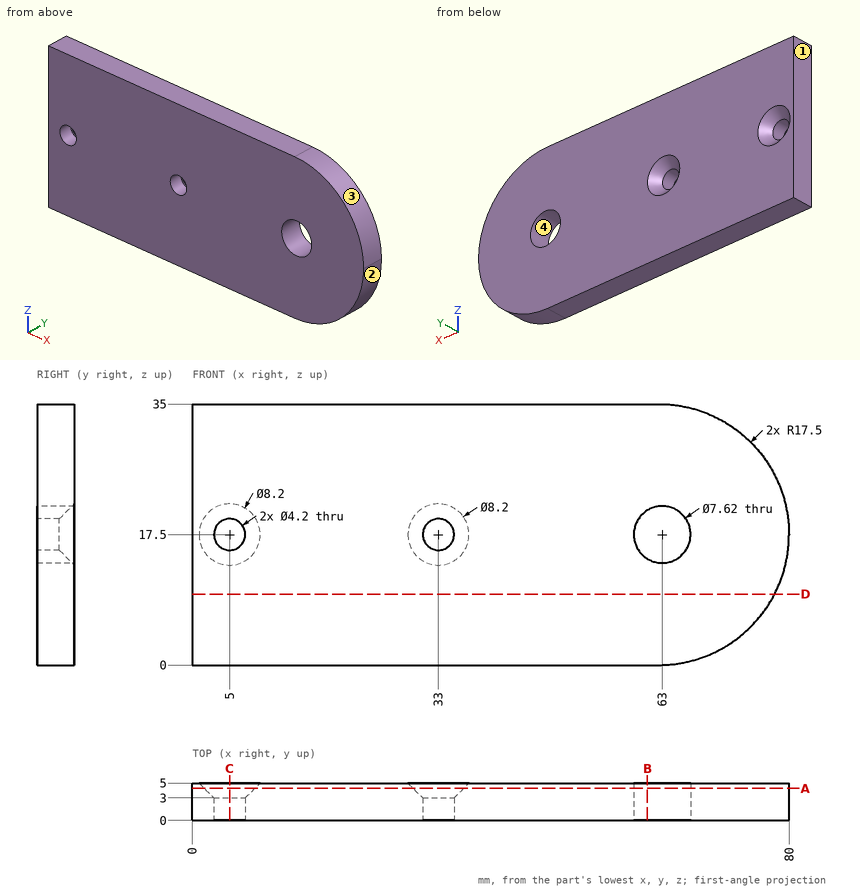
Geometry check sheet. Reference: drawing and pictorial views, mm from the part's lowest x, y, z. Coordinates: 2 decimals unless noted, no trailing zeros. Order: outer loops, then holes, each group sorted by start corner. A loop starts at its lowest first (then second) coordinate and runs counter-clockwise, first axis right, second up. Notation, with made-up numbers: M 4,69 L 57,69 A19 ccw 57,91 Z; hole C 34,57.5 d2. An arc over 180 degrees is marked long. Write each question's results on one line, items separated by ' | '. Start each with the question number.
1. Material ranges on probe 1 along Z at (x, y) = (33, 2.05); probe 2 along X at (y, z) = (3.6, 15.5) (1 decimal); probe 3 along X at (y, z) = (4, 18.5), recorded low to high.
2. Mould release check, pull along Z, two halves, no side actions. Record for the marked faces 1, 2, 3 and 4: +Z half, -Z half, draft (parallel to the pull), parting line (faces both ways), or undercut.
3. Go/stop test with flat-tipped pins: P1, Ø3, axis at y = 3, z = 31, coming from the +X side; P2, Ø4, axis at x = 5, z = 17.5, coming from the +Y side. Record where each tip stops, or that it passes through.
4. Cross-section at A-A on y = 4.3. State how many separate pieces and enclosed holes the cut face has, and give its area (3 significant figures).
5. Cross-section at B-B on x = 61. Record the cut outline in (y, z).
6. Cross-section at C-C on x = 5. Record the cut outline in (y, z), and give its area (3 significant figures).
7. Cross-section at D-D on z = 9.5. Record the cut outline in (x, y).
Checks:
1) probe 1: z = 0 to 15.4, 19.6 to 35 | probe 2: x = 0 to 3.2, 6.8 to 31.2, 34.8 to 59.8, 66.2 to 79.9 | probe 3: x = 0 to 2.07, 7.93 to 30.07, 35.93 to 59.32, 66.68 to 79.97
2) face 1: draft | face 2: -Z half | face 3: +Z half | face 4: undercut
3) P1: stops at x = 75.24 | P2: passes through
4) separate pieces: 1 | enclosed holes: 3 | area: 2,550 mm²
5) outline: M 0,0 L 5,0 L 5,14.26 L 0,14.26 Z; M 0,20.74 L 5,20.74 L 5,35 L 0,35 Z
6) outline: M 0,0 L 5,0 L 5,13.4 L 3,15.4 L 0,15.4 Z; M 0,19.6 L 3,19.6 L 5,21.6 L 5,35 L 0,35 Z | area: 150 mm²
7) outline: M 0,0 L 78.06,0 L 78.06,5 L 0,5 Z
